```python
from build123d import *

# Parameters (mm, degrees)
SKETCH1_W           = 135
SKETCH1_H           = 165
BOSS_EXTRUDE1_DEPTH = 65
SKETCH2_W           = 105
SKETCH2_H           = 135
CUT_EXTRUDE1_DEPTH  = 66
SKETCH3_W           = 30
SKETCH3_H           = 2.27229553
CUT_EXTRUDE2_DEPTH  = 12
SKETCH4_W           = 25
SKETCH4_H           = 4
CUT_EXTRUDE3_DEPTH  = 66
SKETCH5_W           = 115
SKETCH5_H           = 6.5
CUT_EXTRUDE4_DEPTH  = 66
SKETCH7_R           = 5
BOSS_EXTRUDE2_DEPTH = 13
BOSS_EXTRUDE2_TAPER = 3
SKETCH8_R           = 5
BOSS_EXTRUDE3_DEPTH = 13
BOSS_EXTRUDE3_TAPER = 3
SKETCH9_R           = 5
BOSS_EXTRUDE4_DEPTH = 13
BOSS_EXTRUDE4_TAPER = 3
SKETCH10_W          = 105
SKETCH10_H          = 49.956638738
CUT_EXTRUDE5_DEPTH  = 15
CHAMFER3_SIZE       = 3
SKETCH14_W          = 63
SKETCH14_H          = 22
CUT_EXTRUDE6_DEPTH  = 4
SKETCH15_W          = 25
SKETCH15_H          = 25
CUT_EXTRUDE7_DEPTH  = 13


with BuildPart() as part:
    # Sketch1 → Boss-Extrude1 (new body)
    with BuildSketch(Plane(origin=(0, 0, 0), x_dir=(1, 0, 0), z_dir=(0, 1, 0))):
        Rectangle(SKETCH1_W, SKETCH1_H)
    extrude(amount=BOSS_EXTRUDE1_DEPTH)

    # Sketch2 → Cut-Extrude1 (cut, through all)
    with BuildSketch(Plane(origin=(0, 65, 0), x_dir=(1, 0, 0), z_dir=(0, 1, 0))):
        Rectangle(SKETCH2_W, SKETCH2_H)
    extrude(amount=-CUT_EXTRUDE1_DEPTH, mode=Mode.SUBTRACT)

    # Sketch3 → Cut-Extrude2 (cut)
    with BuildSketch(Plane(origin=(-52.5, 0, 0), x_dir=(0, 0, -1), z_dir=(1, 0, 0))):
        with Locations((-27.5, 49)):
            Rectangle(SKETCH3_W, SKETCH3_H)
    extrude(amount=-CUT_EXTRUDE2_DEPTH, mode=Mode.SUBTRACT)

    # Sketch4 → Cut-Extrude3 (cut, through all)
    with BuildSketch(Plane(origin=(0, 65, 0), x_dir=(1, 0, 0), z_dir=(0, 1, 0))):
        with Locations((-32.5, 74.5)):
            Rectangle(SKETCH4_W, SKETCH4_H)
    extrude(amount=-CUT_EXTRUDE3_DEPTH, mode=Mode.SUBTRACT)

    # Sketch5 → Cut-Extrude4 (cut, through all)
    with BuildSketch(Plane(origin=(0, 65, 0), x_dir=(1, 0, 0), z_dir=(0, 1, 0))):
        with Locations((0, -75.5)):
            Rectangle(SKETCH5_W, SKETCH5_H)
    extrude(amount=-CUT_EXTRUDE4_DEPTH, mode=Mode.SUBTRACT)

    # Sketch7 → Boss-Extrude2 (add)
    with BuildSketch(Plane.XZ):
        with Locations((-60, -75)):
            Circle(SKETCH7_R)
    extrude(amount=BOSS_EXTRUDE2_DEPTH, taper=BOSS_EXTRUDE2_TAPER)

    # Sketch8 → Boss-Extrude3 (add)
    with BuildSketch(Plane.XZ):
        with Locations((60, -75)):
            Circle(SKETCH8_R)
    extrude(amount=BOSS_EXTRUDE3_DEPTH, taper=BOSS_EXTRUDE3_TAPER)

    # Sketch9 → Boss-Extrude4 (add)
    with BuildSketch(Plane.XZ):
        with Locations((60, 72.5)):
            Circle(SKETCH9_R)
        with Locations((-60, 73.301994408)):
            Circle(SKETCH9_R)
    extrude(amount=BOSS_EXTRUDE4_DEPTH, taper=BOSS_EXTRUDE4_TAPER)

    # Sketch10 → Cut-Extrude5 (cut)
    with BuildSketch(Plane.XY.offset(82.5)):
        with Locations((0, 33)):
            Rectangle(SKETCH10_W, SKETCH10_H)
    extrude(amount=-CUT_EXTRUDE5_DEPTH, mode=Mode.SUBTRACT)

    # Chamfer3
    chamfer3_edges = [part.edges().sort_by_distance(p)[0] for p in [
        (52.5, 33, 82.5),
        (0, 57.978319369, 82.5),
        (-52.5, 33, 82.5),
        (0, 8.021680631, 82.5),
    ]]
    chamfer(chamfer3_edges, length=CHAMFER3_SIZE)

    # Sketch14 → Cut-Extrude6 (cut)
    with BuildSketch(Plane.XY.offset(-67.5)):
        with Locations((0, 54)):
            Rectangle(SKETCH14_W, SKETCH14_H)
    extrude(amount=-CUT_EXTRUDE6_DEPTH, mode=Mode.SUBTRACT)

    # Sketch15 → Cut-Extrude7 (cut)
    with BuildSketch(Plane.XY.offset(-71.5)):
        with Locations((0, 55.862062237)):
            Rectangle(SKETCH15_W, SKETCH15_H)
    extrude(amount=-CUT_EXTRUDE7_DEPTH, mode=Mode.SUBTRACT)


solid = part.part
```
Geometry check sheet. Reference: the model listing, model coordinates, mm. A direction names the side the tool comes from. Round coordinates to 2 decimals unless told otherwise and drop trailing zeros. Loops run counter-clockwise (first coordinate to the right, second up) from the corner with the lowest first, then second, coordinate; pieces in that order, holes last. Notation, with made-up numbers: (-14.5, 55.5) - (20.5, 55.5) arc R27 ccw to (20.5, 87.5) - close; hole circle Ø10 at (-17, -32.5). An arc over 180 degrees is marked (long way). Write each question's results on one line, items separated by ' | '. Start each with the question number.
Q1. Cross-section at A-A on x = -49. Enter the section's corners in (y, z).
Q2. Thickness scan on line 1 (X direction, y = 21.5, z = 4); line 2 (X direction, y = 58.5, z = 75.5); line 3 (Z direction, x = 11.5, y = 7.5). Record the ranges inside material, lowest first. Write a range as [from, to].
Q3. Access from +Z, -Z, +X, -X, +Y, -Y to the whole of each face (thin tool, end or side, straight path). Record for faces 1 (the flat face through (14, 54, -71.5)), 2 (the flat face through (-60, -13, -75)), 3 (the flat face through (-33, 33, -72.5)), 4 (the flat face through (-1, 8.022, 70)).
Q4. Release check for a two-part mould opening along Z. For faces 5 (the flat face through (0, 3, 82.5)), 6 (the flat face through (-52.5, 33, 3)), 7 (the flat face through (-1, 57.978, 70)) record: +Z half, -Z half, draft (parallel to the pull), parting line (faces both ways), or undercut.
Q5. Cross-section at C-C on y = 11. Enter the section's corners in (x, z).
Q6. Cross-section at D-D on x = -28.5. Enter the section's corners in (y, z).
Q7. Cross-section at B-B on z = -17.5. Enter the section's corners in (x, y).
Q8. Gauge pin test, flat ends, axial feed: P1, Ø9, axis at x = 3.5, z = -78.5, coming from the +Y side; P2, Ø13, axis at x = -57.5, z = 30.5, coming from the -Y side; P3, Ø1, axis at x = 5, y = -1.5, coming from the +Z side; P4, Ø8, axis at y = -3, z = -8.5, coming from the +X side. Record the tip position at first contact, or that the pin passes through.
Answers below:
1) outline: (0, -82.5) - (65, -82.5) - (65, -67.5) - (0, -67.5) - close; (0, 67.5) - (8.02, 67.5) - (8.02, 72.25) - (0, 72.25) - close; (0, 78.75) - (8.02, 78.75) - (8.02, 79.5) - (5.02, 82.5) - (0, 82.5) - close; (57.98, 67.5) - (65, 67.5) - (65, 72.25) - (57.98, 72.25) - close; (57.98, 78.75) - (65, 78.75) - (65, 82.5) - (60.98, 82.5) - (57.98, 79.5) - close
2) line 1: x = [-67.5, -52.5], [52.5, 67.5] | line 2: x = [-67.5, -57.5], [57.5, 67.5] | line 3: z = [-82.5, -67.5], [67.5, 72.25], [78.75, 80.02]
3) face 1: +Y | face 2: +Z, -Z, +X, -X, -Y | face 3: +Y, -Y | face 4: +Z
4) face 5: +Z half | face 6: undercut | face 7: draft
5) outline: (-67.5, -82.5) - (67.5, -82.5) - (67.5, 82.5) - (55.5, 82.5) - (52.5, 79.5) - (52.5, 78.75) - (57.5, 78.75) - (57.5, 72.25) - (52.5, 72.25) - (52.5, -67.5) - (-52.5, -67.5) - (-52.5, 72.25) - (-57.5, 72.25) - (-57.5, 78.75) - (-52.5, 78.75) - (-52.5, 79.5) - (-55.5, 82.5) - (-67.5, 82.5) - close; hole (-45, -76.5) - (-20, -76.5) - (-20, -72.5) - (-45, -72.5) - close
6) outline: (0, -82.5) - (65, -82.5) - (65, -76.5) - (0, -76.5) - close; (0, -72.5) - (65, -72.5) - (65, -71.5) - (43, -71.5) - (43, -67.5) - (0, -67.5) - close; (0, 67.5) - (8.02, 67.5) - (8.02, 72.25) - (0, 72.25) - close; (0, 78.75) - (8.02, 78.75) - (8.02, 79.5) - (5.02, 82.5) - (0, 82.5) - close; (57.98, 67.5) - (65, 67.5) - (65, 72.25) - (57.98, 72.25) - close; (57.98, 78.75) - (65, 78.75) - (65, 82.5) - (60.98, 82.5) - (57.98, 79.5) - close
7) outline: (-67.5, 0) - (-52.5, 0) - (-52.5, 65) - (-67.5, 65) - close; (52.5, 0) - (67.5, 0) - (67.5, 65) - (52.5, 65) - close
8) P1: stops at y = 43.36 | P2: stops at y = 0 | P3: passes through | P4: stops at x = 67.5
